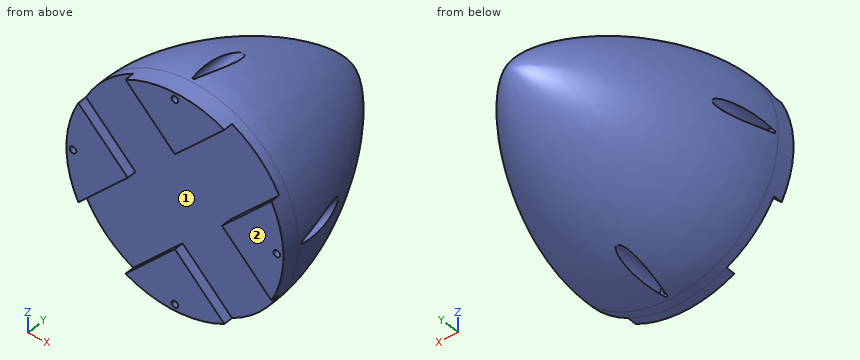
from build123d import *

# Parameters (mm, degrees)
SKETCH3_R           = 57.5
BOSS_EXTRUDE1_DEPTH = 5
BOSS_EXTRUDE2_DEPTH = 5
CIRPATTERN2_COUNT   = 4
SKETCH7_R           = 1.75
CUT_EXTRUDE1_DEPTH  = 12
SKETCH8_R           = 3.5
CUT_EXTRUDE2_DEPTH  = 102.62602644
CIRPATTERN1_COUNT   = 4


with BuildPart() as part:
    # Sketch1 → Revolve2 (revolve)
    with BuildSketch(Plane.XY):
        with BuildLine():
            Line((47.5, 0), (57.5, 0))
            add(Edge.make_bspline(
                [(57.5, 0), (57.5, 22.486866931), (44.523412509, 66.822797193), (11.090180384, 103.62602634), (0, 103.62602634)],
                knots=[0, 0, 0, 0, 0, 1, 1, 1, 1, 1], degree=4))
            Line((0, 103.62602634), (0, 93.62602634))
            add(Edge.make_bspline(
                [(47.5, 0), (47.5, 22.486866931), (34.523412509, 66.822797193), (10.174500673, 93.62602634), (0, 93.62602634)],
                knots=[0, 0, 0, 0, 0, 1, 1, 1, 1, 1], degree=4))
        make_face()
    revolve(axis=Axis((0, 0, 0), (0, 1, 0)))

    # Sketch3 → Boss-Extrude1 (add)
    with BuildSketch(Plane.XZ):
        Circle(SKETCH3_R)
    extrude(amount=BOSS_EXTRUDE1_DEPTH)

    # Sketch9 → Boss-Extrude2 (add)
    with BuildSketch(Plane.XZ.offset(5)):
        with BuildLine():
            Line((0, -25), (-26.189468851, -51.189468851))
            ThreePointArc((-26.189468851, -51.189468851), (0, -57.5), (26.189468851, -51.189468851))
            Line((26.189468851, -51.189468851), (0, -25))
        make_face()
    boss_extrude2 = extrude(amount=BOSS_EXTRUDE2_DEPTH)

    # CirPattern2: Boss-Extrude2 ×4 about axis
    cirpattern2_axis = Axis((0, 0, 0), (0, 1, 0))
    for i in range(1, CIRPATTERN2_COUNT):
        add(boss_extrude2.rotate(cirpattern2_axis, i * 360 / CIRPATTERN2_COUNT))

    # Sketch7 → Cut-Extrude1 (cut)
    with BuildSketch(Plane.XZ.offset(10)):
        with Locations((-54, 0)):
            Circle(SKETCH7_R)
    cut_extrude1 = extrude(amount=-CUT_EXTRUDE1_DEPTH, mode=Mode.SUBTRACT)

    # Sketch8 → Cut-Extrude2 (cut, through all)
    with BuildSketch(Plane.XZ.offset(-2)):
        with Locations((-54, 0)):
            Circle(SKETCH8_R)
    cut_extrude2 = extrude(amount=-CUT_EXTRUDE2_DEPTH, mode=Mode.SUBTRACT)

    # CirPattern1: Cut-Extrude1, Cut-Extrude2 ×4 about axis
    cirpattern1_axis = Axis((0, 0, 0), (0, 1, 0))
    for i in range(1, CIRPATTERN1_COUNT):
        add(cut_extrude1.rotate(cirpattern1_axis, i * 360 / CIRPATTERN1_COUNT), mode=Mode.SUBTRACT)
        add(cut_extrude2.rotate(cirpattern1_axis, i * 360 / CIRPATTERN1_COUNT), mode=Mode.SUBTRACT)


solid = part.part
For this review, take the finished solid that the model builds, in its own axes (mm). Face numbers are marked on the shaded views. A direction names the side the tool comes from. Give positions to 0.01 mm unless a question says otherwise; leave off trailing zeros. Use CSV: the item, a comma, the result in double quotes.
Q1. Tool access review of the marked faces 1 and 2: name each direction out of +Z, -Z, +X, -X, +Y, -Y from which nothing blocks a thin tool from reaching the whole face with its end or side.
Conclusion:
face 1,"-Y"
face 2,"+Z, -Z, +X, -X, -Y"
Q2. For P1, Ø4, axis at x = 36.5, z = 45, coming from the -Y side; P2, Ø3.5, axis at x = -1, z = -54.5, coming from the +Y side; P3, Ø1.5, axis at y = 32, z = -9, coming from the +X side; P4, Ø3, axis at x = 54, z = 0, coming from the +Y side, all flat-tipped, find the tip position at first contact; note any pin that passes through.
Conclusion:
P1,"y = -5"
P2,"y = 2"
P3,"x = 50.84"
P4,"through"
Q3. To check wall thickness, follow probe 1 along Y at (x, z) = (12, 10); probe 2 along Y at (x, z) = (6.5, -9); probe 3 along X at (y, z) = (51.5, -27). State the ranges of each line that lie inside material, in increasing order. Write a range as [from, to].
Conclusion:
probe 1,"[-5, 0], [82.42, 93.09]"
probe 2,"[-5, 0], [87.22, 97.4]"
probe 3,"[-34.04, -21.31], [21.31, 34.04]"
